Design review of the part built by this model. Coordinates are the model's own, in mm. Face numbers are marked on the shaded views. A direction names the side the tool comes from. Round coordinates to 2 decimals unless told otherwise and drop trailing zeros. Order: outer loops, then holes, each group sorted by start corner. A loop starts at its lowest first (then second) coordinate and runs counter-clockwise, first axis right, second up. Notation, with made-up numbers: (70, 0.25) - (115, 0.25) arc R17 ccw to (115, 30.25) - close; hole circle Ø10 at (18, -34.5). An arc over 180 degrees is marked (long way). Answer as a JSON object with one key per item and string values. Group by question number.
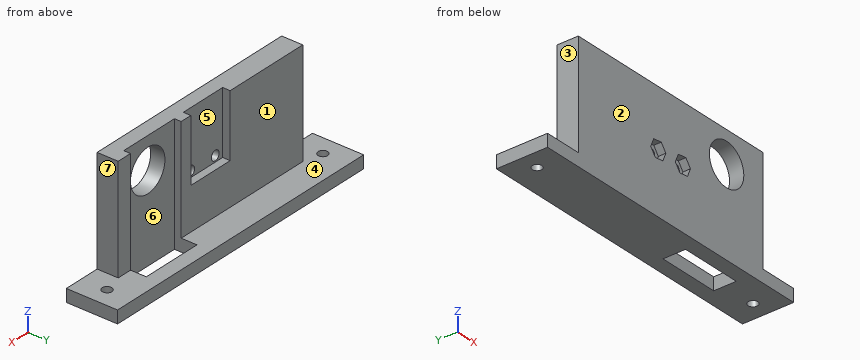
from build123d import *

# Parameters (mm, degrees)
SKETCH1_W                 = 75
SKETCH1_H                 = 16.798090687
SKETCH1_H_2               = 35
BODY_DEPTH                = 7
SKETCH3_W                 = 16
SKETCH3_H                 = 21
CHIP_DIVET_DEPTH          = 2.5
SKETCH4_R                 = 1.6
CHIP_MOUNTING_HOLES_DEPTH = 58.827758025
CHIP_CAPTIVE_NUTS_DEPTH   = 2.5
SKETCH6_R                 = 7
ROUTING_HOLE_DEPTH        = 59.075809062
SKETCH7_W                 = 100
SKETCH7_H                 = 4.201909313
FACE_PLATE_DEPTH          = 10
SKETCH8_W                 = 20.6
SKETCH8_H                 = 7.5
SWITCH_HOLE_DEPTH         = 66.770735847
SKETCH2_R                 = 1.6
MOUNTING_HOLES_DEPTH      = 66.770735847


with BuildPart() as part:
    # Sketch1 → body (new body)
    with BuildSketch(Plane(origin=(0, 0, 0), x_dir=(1, 0, 0), z_dir=(0, 1, 0))):
        Polygon((-50, 6.298090687), (-37.5, 6.298090687), (37.5, 6.298090687), (50, 6.298090687), (50, 10.5), (-50, 10.5), align=None)
        with Locations((0, -2.100954656)):
            Rectangle(SKETCH1_W, SKETCH1_H)
        with Locations((0, -11.201909313)):
            Rectangle(SKETCH1_W, SKETCH1_H_2)
    extrude(amount=BODY_DEPTH)

    # Sketch3 → chip-divet (cut)
    with BuildSketch(Plane(origin=(0, 7, 0), x_dir=(1, 0, 0), z_dir=(0, 1, 0))):
        with Locations((0, -18.201909313)):
            Rectangle(SKETCH3_W, SKETCH3_H)
    extrude(amount=-CHIP_DIVET_DEPTH, mode=Mode.SUBTRACT)

    # Sketch4 → chip-mounting-holes (cut, through all)
    with BuildSketch(Plane(origin=(0, 4.5, 0), x_dir=(1, 0, 0), z_dir=(0, 1, 0))):
        with Locations(Location((-5, -9.701909313, 0), (0, 0, 270))):
            Circle(SKETCH4_R)
        with Locations(Location((5, -9.701909313, 0), (0, 0, 270))):
            Circle(SKETCH4_R)
    extrude(amount=-CHIP_MOUNTING_HOLES_DEPTH, mode=Mode.SUBTRACT)

    # Sketch5 → chip-captive-nuts (cut)
    with BuildSketch(Plane.XZ):
        Polygon((6.21170825, 12.555286806), (3.13475673, 12.177968186), (1.92304848, 9.324590694), (3.78829175, 6.848531821), (6.86524327, 7.22585044), (8.07695152, 10.079227933), align=None)
        Polygon((-3.78829175, 12.555286806), (-6.86524327, 12.177968186), (-8.07695152, 9.324590694), (-6.21170825, 6.848531821), (-3.13475673, 7.22585044), (-1.92304848, 10.079227933), align=None)
    extrude(amount=-CHIP_CAPTIVE_NUTS_DEPTH, mode=Mode.SUBTRACT)

    # Sketch6 → routing-hole (cut, through all)
    with BuildSketch(Plane(origin=(0, 7, 0), x_dir=(1, 0, 0), z_dir=(0, 1, 0))):
        with Locations(Location((22.75, -18.201909313, 0), (0, 0, 270))):
            Circle(SKETCH6_R)
    extrude(amount=-ROUTING_HOLE_DEPTH, mode=Mode.SUBTRACT)

    # Sketch7 → face-plate (add)
    with BuildSketch(Plane(origin=(0, 7, 0), x_dir=(1, 0, 0), z_dir=(0, 1, 0))):
        with Locations((0, 8.399045343)):
            Rectangle(SKETCH7_W, SKETCH7_H)
    extrude(amount=FACE_PLATE_DEPTH)

    # Sketch8 → switch-hole (cut, through all)
    with BuildSketch(Plane(origin=(0, 0, -10.5), x_dir=(-1, 0, 0), z_dir=(0, 0, -1))):
        with Locations((-22.2, 8.5)):
            Rectangle(SKETCH8_W, SKETCH8_H)
    extrude(amount=-SWITCH_HOLE_DEPTH, mode=Mode.SUBTRACT)

    # Sketch2 → mounting-holes (cut, through all)
    with BuildSketch(Plane(origin=(0, 0, -10.5), x_dir=(-1, 0, 0), z_dir=(0, 0, -1))):
        with Locations((-43.86, 8.5)):
            Circle(SKETCH2_R)
        with Locations((43.86, 8.5)):
            Circle(SKETCH2_R)
    extrude(amount=-MOUNTING_HOLES_DEPTH, mode=Mode.SUBTRACT)


solid = part.part
1. Take a section at A-A, the plane y = 8.5. Give the boundary of the cut face in (x, z), then the cut area to 3 significant figures.
2. Take a section at C-C, the plane x = 19. Give the boundary of the cut face in (y, z).
3. Take a section at B-B, the plane x = 43.86. Give the boundary of the cut face in (y, z).
4. To check wall thickness, follow line 1 (X direction, y = 6.25, z = 27.5); line 2 (Y direction, x = 43.86, z = -7.9); line 3 (X direction, y = 6.5, z = 0.5). State the ranges of each line that lie inside material, in increasing order. Write a range as from..to.
5. Mouldability with a two-part tool opening along X and no side actions: class the marked faces 4, 5, 6 and 7 as pulls with the +X half, pulls with the -X half, needs draft (parallel to the pull), parting line crosses it, or undercut.
6. Tool access review of the marked faces 1, 2 and 3: name each direction out of +Z, -Z, +X, -X, +Y, -Y from which nothing blocks a thin tool from reaching the whole face with its end or side.
7. Take a section at D-D, the plane z = 19.5. Give the boundary of the cut face in (x, y).
8. Clearance check with flat-ended pins moving along their axes: P1, Ø2, axis at y = 3.5, z = 15.5, coming from the +X side; P2, Ø3, axis at x = -14.5, z = 11.5, coming from the +Y side; P3, Ø11, axis at x = 22.75, z = 18.2, coming from the -Y side; P4, Ø8, axis at x = -0.5, z = 21, coming from the +Y side. State where each tip first meets the part, or that it passes through.
Response values:
{
 "1": {"outline": "(-50, -10.5) - (-45.46, -10.5) - (-45.46, -6.3) - (-50, -6.3) - close; (-42.26, -10.5) - (11.9, -10.5) - (11.9, -6.3) - (-42.26, -6.3) - close; (32.5, -10.5) - (42.26, -10.5) - (42.26, -6.3) - (32.5, -6.3) - close; (45.46, -10.5) - (50, -10.5) - (50, -6.3) - (45.46, -6.3) - close", "area": "307 mm2"},
 "2": {"outline": "(0, -10.5) - (4.75, -10.5) - (4.75, 12.29) - (0, 12.29) - close; (0, 24.11) - (4.75, 24.11) - (4.75, 28.7) - (0, 28.7) - close; (12.25, -10.5) - (17, -10.5) - (17, -6.3) - (12.25, -6.3) - close"},
 "3": {"outline": "(0, -10.5) - (6.9, -10.5) - (6.9, -6.3) - (0, -6.3) - close; (10.1, -10.5) - (17, -10.5) - (17, -6.3) - (10.1, -6.3) - close"},
 "4": {"line 1": "-37.5..-8, 8..11.9, 32.5..37.5", "line 2": "0..6.9, 10.1..17", "line 3": "-37.5..11.9, 32.5..37.5"},
 "5": {"face 4": "needs draft", "face 5": "undercut", "face 6": "undercut", "face 7": "pulls with the +X half"},
 "6": {"face 1": "+Z, +X, -X, +Y", "face 2": "+Z, -Z, +X, -X, -Y", "face 3": "+Z, -X, +Y, -Y"},
 "7": {"outline": "(-37.5, 0) - (15.87, 0) - (15.87, 4.75) - (11.9, 4.75) - (11.9, 7) - (8, 7) - (8, 4.5) - (-8, 4.5) - (-8, 7) - (-37.5, 7) - close; (29.63, 0) - (37.5, 0) - (37.5, 7) - (32.5, 7) - (32.5, 4.75) - (29.63, 4.75) - close"},
 "8": {"P1": "x = 37.5", "P2": "y = 7", "P3": "through", "P4": "y = 4.5"}
}
